Check sheet for the modelled part. Datum: model origin and axes. Units: mm. Face numbers are marked on the shaded views. A direction names the side the tool comes from. Coordinates: 2 decimals unless noted, no trailing zeros. Loops run counter-clockwise (first coordinate to the right, second up) from the corner with the lowest first, then second, coordinate; pieces in that order, holes last. Notation, with made-up numbers: M -24.75,-35.5 L -5.75,-35.5 A4 ccw -5.75,-28.5 Z; hole C -3.5,78 d7. An arc over 180 degrees is marked long. Use CSV: the item, a comma, the result in double quotes. Start each with the question number.
(1) Section check A-A on z = 0.25. Give the number of separate pieces and of enclosed holes in the cut face, and give its area (3 significant figures).
(2) Go/stop test with flat-tipped pins: pin 1 Ø8 at (x, z) = (-45, 8) entering from +Y; pin 2 Ø5 at (x, y) = (226, -3.5) entering from +Z; pin 3 Ø6 at (y, z) = (6, 5) entering from -X. Record where each tip stops, or that it passes through.
(3) Scan lines: line 1 (Y direction, x = 161, z = -9); line 2 (Y direction, x = 87.5, z = 7.75); line 3 (Y direction, x = 199, z = 10.25). Record each from-to range of solid material in increasing order.
(4) Section check B-B on x = -33. Record the cut outline in (y, z), and give its area (3 significant figures).
(5) Set-up check for the marked faces 1, 2 and 3: record each of +Z, -Z, +X, -X, +Y, -Y from which the full face is reachable in a straight line by a thin tool's end or side.
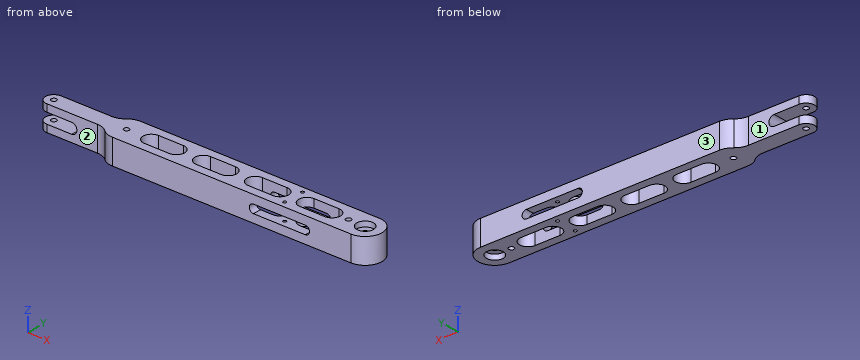
from build123d import *

# Parameters (mm, degrees)
SKETCH1_R               = 2.5
BOSS_EXTRUDE1_DEPTH     = 12
CUT_EXTRUDE1_REACH      = 249.459
CUT_EXTRUDE3_REACH      = 249.685
LPATTERN1_COUNT         = 4
LPATTERN1_PITCH         = 50
CUT_EXTRUDE4_REACH      = 249.685
SKETCH5_R               = 2.5
SKETCH6_R               = 8
CUT_EXTRUDE5_DEPTH      = 5
CUT_EXTRUDE7_DEPTH      = 248.459087528
CUT_EXTRUDE7_DEPTH_BACK = 248.459087528
SKETCH9_R               = 1.5
CUT_EXTRUDE8_DEPTH      = 248.685284181


with BuildPart() as part:
    # Sketch1 → Boss-Extrude1 (new, symmetric)
    with BuildSketch(Plane.XY):
        with BuildLine():
            Line((0, 16), (230, 16))
            ThreePointArc((230, 16), (246, 0), (230, -16))
            Line((230, -16), (0, -16))
            ThreePointArc((0, -16), (-5.656854249, -14.966629547), (-10.583005244, -12))
            ThreePointArc((-10.583005244, -12), (-15.509156239, -9.033370453), (-21.166010489, -8))
            Line((-21.166010489, -8), (-70, -8))
            ThreePointArc((-70, -8), (-78, 0), (-70, 8))
            Line((-70, 8), (-21.166010489, 8))
            ThreePointArc((-21.166010489, 8), (-15.509156239, 9.033370453), (-10.583005244, 12))
            ThreePointArc((-10.583005244, 12), (-5.656854249, 14.966629547), (0, 16))
        make_face()
        Circle(SKETCH1_R, mode=Mode.SUBTRACT)
        with Locations((-70, 0)):
            Circle(SKETCH1_R, mode=Mode.SUBTRACT)
    extrude(amount=BOSS_EXTRUDE1_DEPTH, both=True)

    # Sketch2 → Cut-Extrude1 (cut, up to next)
    with BuildSketch(Plane.XZ.offset(8), mode=Mode.PRIVATE) as cut_extrude1_sk1:
        with BuildLine():
            Line((-78, -5), (-46, -5))
            ThreePointArc((-46, -5), (-41, 0), (-46, 5))
            Line((-46, 5), (-78, 5))
            Line((-78, 5), (-78, -5))
        make_face()
    cut_extrude1_tool1 = extrude(cut_extrude1_sk1.sketch, amount=-CUT_EXTRUDE1_REACH, mode=Mode.PRIVATE) & part.part
    add(cut_extrude1_tool1.solids().sort_by_distance((-60.019172, -8, 0))[0], mode=Mode.SUBTRACT)

    # Sketch4 → Cut-Extrude3 (cut, up to next)
    with BuildSketch(Plane.XY.offset(12), mode=Mode.PRIVATE) as cut_extrude3_sk1:
        with BuildLine():
            Line((24, 8), (48, 8))
            ThreePointArc((48, 8), (56, 0), (48, -8))
            Line((48, -8), (24, -8))
            ThreePointArc((24, -8), (16, 0), (24, 8))
        make_face()
    cut_extrude3_tool1 = extrude(cut_extrude3_sk1.sketch, amount=-CUT_EXTRUDE3_REACH, mode=Mode.PRIVATE) & part.part
    cut_extrude3 = cut_extrude3_tool1.solids().sort_by_distance((36, 0, 12))[0]
    add(cut_extrude3, mode=Mode.SUBTRACT)

    # LPattern1: Cut-Extrude3 ×4
    with Locations(*[(i * LPATTERN1_PITCH, 0, 0) for i in range(1, LPATTERN1_COUNT)]):
        add(cut_extrude3, mode=Mode.SUBTRACT)

    # Sketch5 → Cut-Extrude4 (cut, up to next)
    with BuildSketch(Plane.XY.offset(12), mode=Mode.PRIVATE) as cut_extrude4_sk1:
        with Locations((230, 0)):
            Circle(SKETCH5_R)
    cut_extrude4_tool1 = extrude(cut_extrude4_sk1.sketch, amount=-CUT_EXTRUDE4_REACH, mode=Mode.PRIVATE) & part.part
    # Sketch5 → Cut-Extrude4 (cut, up to next)
    with BuildSketch(Plane.XY.offset(12), mode=Mode.PRIVATE) as cut_extrude4_sk2:
        with Locations((214, 0)):
            Circle(SKETCH5_R)
    cut_extrude4_tool2 = extrude(cut_extrude4_sk2.sketch, amount=-CUT_EXTRUDE4_REACH, mode=Mode.PRIVATE) & part.part
    add(cut_extrude4_tool1.solids().sort_by_distance((230, 0, 12))[0], mode=Mode.SUBTRACT)
    add(cut_extrude4_tool2.solids().sort_by_distance((214, 0, 12))[0], mode=Mode.SUBTRACT)

    # Sketch6 → Cut-Extrude5 (cut)
    with BuildSketch(Plane.XY.offset(12)):
        with Locations((230, 0)):
            Circle(SKETCH6_R)
    cut_extrude5 = extrude(amount=-CUT_EXTRUDE5_DEPTH, mode=Mode.SUBTRACT)

    # Mirror1: Cut-Extrude5 across plane
    add(cut_extrude5.mirror(Plane.XY), mode=Mode.SUBTRACT)

    # Sketch8 → Cut-Extrude7 (cut, two sides: drawn at the far end of the back side and taken through both)
    with BuildSketch(Plane(origin=(0, -8, 0), x_dir=(1, 0, 0), z_dir=(0, 1, 0)).offset(-CUT_EXTRUDE7_DEPTH_BACK)):
        with BuildLine():
            Line((136, 4), (186, 4))
            ThreePointArc((186, 4), (190, 0), (186, -4))
            Line((186, -4), (136, -4))
            ThreePointArc((136, -4), (132, 0), (136, 4))
        make_face()
    extrude(amount=CUT_EXTRUDE7_DEPTH + CUT_EXTRUDE7_DEPTH_BACK, mode=Mode.SUBTRACT)

    # Sketch9 → Cut-Extrude8 (cut, through all)
    with BuildSketch(Plane.XY.offset(12)):
        with Locations((161, 10)):
            Circle(SKETCH9_R)
        with Locations((161, -10)):
            Circle(SKETCH9_R)
    extrude(amount=-CUT_EXTRUDE8_DEPTH, mode=Mode.SUBTRACT)


solid = part.part
Outcome:
1,separate pieces,"2"
1,enclosed holes,"5"
1,area,"5,050 mm²"
2,pin 1,"stops at y = 8"
2,pin 2,"stops at z = 7"
2,pin 3,"stops at x = -77.42"
3,line 1,"y = -16 to -11.5, -8.5 to 8.5, 11.5 to 16"
3,line 2,"y = -16 to -8, 8 to 16"
3,line 3,"y = -16 to -7.94, 7.94 to 16"
4,outline,"M -8,-12 L 8,-12 L 8,12 L -8,12 Z"
4,area,"384 mm²"
5,face 1,"+Z, -Z, -X, +Y"
5,face 2,"+Z, -Z, -X, -Y"
5,face 3,"+Z, -Z, +X, -X, +Y"
